from build123d import *

# Parameters (mm, degrees)
SKETCH014_W     = 75.4
SKETCH014_H     = 100
PAD008_DEPTH    = 9
SKETCH015_W     = 71.4
SKETCH015_H     = 96
POCKET006_DEPTH = 7
SKETCH016_W     = 2
SKETCH016_H     = 21.2
SKETCH016_W_2   = 7.2
SKETCH016_H_2   = 2
PAD009_DEPTH    = 5.4
SKETCH017_W     = 20
SKETCH017_H     = 2
POCKET007_DEPTH = 75.401
SKETCH018_R     = 1.6
PAD010_DEPTH    = 10.6
SKETCH019_R     = 3
POCKET008_DEPTH = 2.6
FILLET006_R     = 1
FILLET007_R     = 6
FILLET008_R     = 4
FILLET009_R     = 8
FILLET010_R     = 2


with BuildPart() as part:
    # Sketch014 → Pad008 (new body)
    with BuildSketch(Plane.XY):
        with Locations((0, -28.5)):
            Rectangle(SKETCH014_W, SKETCH014_H)
    extrude(amount=-PAD008_DEPTH)

    # Sketch015 (on Face5 of Pad008) → Pocket006 (cut)
    with BuildSketch(Plane.XY):
        with Locations((0, -28.5)):
            Rectangle(SKETCH015_W, SKETCH015_H)
    extrude(amount=-POCKET006_DEPTH, mode=Mode.SUBTRACT)

    # Sketch016 (on Face4 of Pocket006) → Pad009 (join)
    with BuildSketch(Plane.XY):
        with Locations((-36.7, 0)):
            Rectangle(SKETCH016_W, SKETCH016_H)
        with Locations((36.7, 0)):
            Rectangle(SKETCH016_W, SKETCH016_H)
        with Locations((-22, 20.5)):
            Rectangle(SKETCH016_W_2, SKETCH016_H_2)
    extrude(amount=PAD009_DEPTH)

    # Sketch017 (on Face3 of Pad009) → Pocket007 (cut, through all)
    with BuildSketch(Plane.YZ.offset(37.7)):
        with Locations((-46.5, -5.8)):
            Rectangle(SKETCH017_W, SKETCH017_H)
        with Locations((1.5, -5.8)):
            Rectangle(SKETCH017_W, SKETCH017_H)
    extrude(amount=-POCKET007_DEPTH, mode=Mode.SUBTRACT)

    # Sketch018 (on Face42 of Pocket007) → Pad010 (join)
    with BuildSketch(Plane.XY.offset(-7)):
        with BuildLine():
            Line((-31.85, 12.1), (-35.7, 12.1))
            Line((-35.7, 12.1), (-35.7, 19.5))
            Line((-35.7, 19.5), (-28.563923, 19.5))
            Line((-28.563923, 19.5), (-28.563923, 14.627247))
            ThreePointArc((-31.85, 12.1), (-29.777243, 12.804879), (-28.563923, 14.627247))
        make_face()
        with Locations((-31.85, 15.5)):
            Circle(SKETCH018_R, mode=Mode.SUBTRACT)
        with BuildLine():
            Line((28.45, 19.5), (35.7, 19.5))
            Line((35.7, 19.5), (35.7, 12.1))
            Line((35.7, 12.1), (31.85, 12.1))
            ThreePointArc((28.45, 15.5), (29.445837, 13.095837), (31.85, 12.1))
            Line((28.45, 19.5), (28.45, 15.5))
        make_face()
        with Locations((31.85, 15.5)):
            Circle(SKETCH018_R, mode=Mode.SUBTRACT)
        with BuildLine():
            Line((35.7, -69.1), (35.7, -76.5))
            Line((35.7, -76.5), (28.45, -76.5))
            Line((28.45, -76.5), (28.45, -72.5))
            ThreePointArc((31.85, -69.1), (29.445837, -70.095837), (28.45, -72.5))
            Line((35.7, -69.1), (31.85, -69.1))
        make_face()
        with Locations((31.85, -72.5)):
            Circle(SKETCH018_R, mode=Mode.SUBTRACT)
        with BuildLine():
            Line((-35.7, -76.5), (-28.45, -76.5))
            Line((-28.45, -76.5), (-28.45, -72.5))
            ThreePointArc((-28.45, -72.5), (-29.445837, -70.095837), (-31.85, -69.1))
            Line((-35.7, -69.1), (-31.85, -69.1))
            Line((-35.7, -76.5), (-35.7, -69.1))
        make_face()
        with Locations((-31.85, -72.5)):
            Circle(SKETCH018_R, mode=Mode.SUBTRACT)
    extrude(amount=PAD010_DEPTH)

    # Sketch019 (on Face7 of Pad010) → Pocket008 (cut)
    with BuildSketch(Plane(origin=(0, 0, -9), x_dir=(1, 0, 0), z_dir=(0, 0, -1))):
        with Locations((-31.85, 72.5)):
            Circle(SKETCH019_R)
        with Locations((31.85, 72.5)):
            Circle(SKETCH019_R)
        with Locations((-31.85, -15.5)):
            Circle(SKETCH019_R)
        with Locations((31.85, -15.5)):
            Circle(SKETCH019_R)
    extrude(amount=-POCKET008_DEPTH, mode=Mode.SUBTRACT)

    # Fillet006
    fillet006_edges = [part.edges().sort_by_distance(p)[0] for p in [
        (-35.7, 19.5, 1.8),
        (35.7, 19.5, 1.8),
    ]]
    fillet(fillet006_edges, radius=FILLET006_R)

    # Fillet007
    fillet007_edges = [part.edges().sort_by_distance(p)[0] for p in [
        (35.7, -76.5, 1.8),
        (-35.7, -76.5, 1.8),
    ]]
    fillet(fillet007_edges, radius=FILLET007_R)

    # Fillet008
    fillet008_edges = [part.edges().sort_by_distance(p)[0] for p in [
        (-37.7, 21.5, -4.5),
        (37.7, 21.5, -4.5),
    ]]
    fillet(fillet008_edges, radius=FILLET008_R)

    # Fillet009
    fillet009_edges = [part.edges().sort_by_distance(p)[0] for p in [
        (-37.7, -78.5, -4.5),
        (37.7, -78.5, -4.5),
    ]]
    fillet(fillet009_edges, radius=FILLET009_R)

    # Fillet010
    fillet010_edges = [part.edges().sort_by_distance(p)[0] for p in [
        (-37.7, -26.5, -9),
        (-36.528427, 20.328427, -9),
        (0, 21.5, -9),
        (36.528427, 20.328427, -9),
        (37.7, -26.5, -9),
        (35.356854, -76.156854, -9),
        (0, -78.5, -9),
        (-35.356854, -76.156854, -9),
    ]]
    fillet(fillet010_edges, radius=FILLET010_R)


with BuildPart() as part_1:
    # Body004 placement: moved
    add(part.part.moved(Location((0, 0, -2))))


solid = part_1.part
Verification items for the finished model (mm, model axes). A direction names the side the tool comes from. Coordinates: 2 decimals unless noted, no trailing zeros. Order: outer loops, then holes, each group sorted by start corner. A loop starts at its lowest first (then second) coordinate and runs counter-clockwise, first axis right, second up. Notation, with made-up numbers: M 34.25,3.25 L 50.25,3.25 A17 ccw 50.25,12.25 Z; hole C 9,-35.5 d9. An arc over 180 degrees is marked long. Write each question's results on one line, items separated by ' | '.
1) Section check C-C on x = 15.5. Record the cut outline in (y, z).
Solved:
outline: M -78.5,-9 A2 ccw -76.5,-11 L 19.5,-11 A2 ccw 21.5,-9 L 21.5,-2 L 19.5,-2 L 19.5,-9 L -76.5,-9 L -76.5,-2 L -78.5,-2 Z
2) Scan lines: line 1 along Y through (x, z) = (6.5, -6.75); line 2 along X through (y, z) = (1, -1.75); line 3 along X through (y, z) = (15.5, -0.75). Record each from-to range of solid material in increasing order. Write a range as [from, to].
Solved:
line 1: y = [-78.5, -76.5], [19.5, 21.5] | line 2: x = [-37.7, -35.7], [35.7, 37.7] | line 3: x = [-35.7, -33.45], [-30.25, -28.56], [28.45, 30.25], [33.45, 35.7]
3) Section check D-D on y = -49.5. Record the cut outline in (x, z), plus the area to 3 significant figures.
Solved:
outline: M -37.7,-9 A2 ccw -35.7,-11 L 35.7,-11 A2 ccw 37.7,-9 L 37.7,-8.8 L 35.7,-8.8 L 35.7,-9 L -35.7,-9 L -35.7,-8.8 L -37.7,-8.8 Z; M -37.7,-6.8 L -35.7,-6.8 L -35.7,-2 L -37.7,-2 Z; M 35.7,-6.8 L 37.7,-6.8 L 37.7,-2 L 35.7,-2 Z | area: 169 mm²
4) Release check for a two-part mould opening along Y. For faces 1 (the face through (37, -10.6, 1)), 2 (the face through (36.559, 20.297, -5.549)), 3 (the face through (0, 19.5, -5)) record: pulls with the +Y half, pulls with the -Y half, needs draft (parallel to the pull), parting line crosses it, or undercut.
Solved:
face 1: pulls with the -Y half | face 2: pulls with the +Y half | face 3: undercut
5) Section check A-A on y = -7. Record the cut outline in (x, z).
Solved:
outline: M -37.7,-9 A2 ccw -35.7,-11 L 35.7,-11 A2 ccw 37.7,-9 L 37.7,-8.8 L 35.7,-8.8 L 35.7,-9 L -35.7,-9 L -35.7,-8.8 L -37.7,-8.8 Z; M -37.7,-6.8 L -35.7,-6.8 L -35.7,3.4 L -37.7,3.4 Z; M 35.7,-6.8 L 37.7,-6.8 L 37.7,3.4 L 35.7,3.4 Z
6) Access from +Z, -Z, +X, -X, +Y, -Y to the whole of each face (thin tool, end or side, straight path). Record for faces 4 (the face through (0, -76.5, -5)), 5 (the face through (-37, -10.6, 1)), 6 (the face through (37, 10.6, 1)).
Solved:
face 4: +Z | face 5: +Z, +X, -X, -Y | face 6: +Z, +X, -X, +Y
7) Gauge pin test, flat ends, axial feed: pin 1 Ø0.6 at (x, y) = (36.5, -51) entering from -Z; pin 2 Ø3.5 at (x, y) = (-33, 14) entering from +Z; pin 3 Ø0.6 at (y, z) = (20, 0.5) entering from -X; pin 4 Ø5 at (x, z) = (0, 1.5) entering from +Y. Record the tip position at first contact, or that the pin passes through.
Solved:
pin 1: stops at z = -10.94 | pin 2: stops at z = 1.6 | pin 3: stops at x = -25.6 | pin 4: passes through
8) Section check B-B on z = -3.75. Record the cut outline in (x, y), plus the area to 3 significant figures.
Solved:
outline: M -37.7,-70.5 A8 ccw -29.7,-78.5 L 29.7,-78.5 A8 ccw 37.7,-70.5 L 37.7,17.5 A4 ccw 33.7,21.5 L -33.7,21.5 A4 ccw -37.7,17.5 Z; hole M -35.7,-69.1 L -31.85,-69.1 A3.4 cw -28.45,-72.5 L -28.45,-76.5 L 28.45,-76.5 L 28.45,-72.5 A3.4 cw 31.85,-69.1 L 35.7,-69.1 L 35.7,12.1 L 31.85,12.1 A3.4 cw 28.45,15.5 L 28.45,19.5 L -28.56,19.5 L -28.56,14.63 A3.4 cw -31.85,12.1 L -35.7,12.1 Z; hole C -31.85,-72.5 d3.2; hole C -31.85,15.5 d3.2; hole C 31.85,-72.5 d3.2; hole C 31.85,15.5 d3.2 | area: 823 mm²
